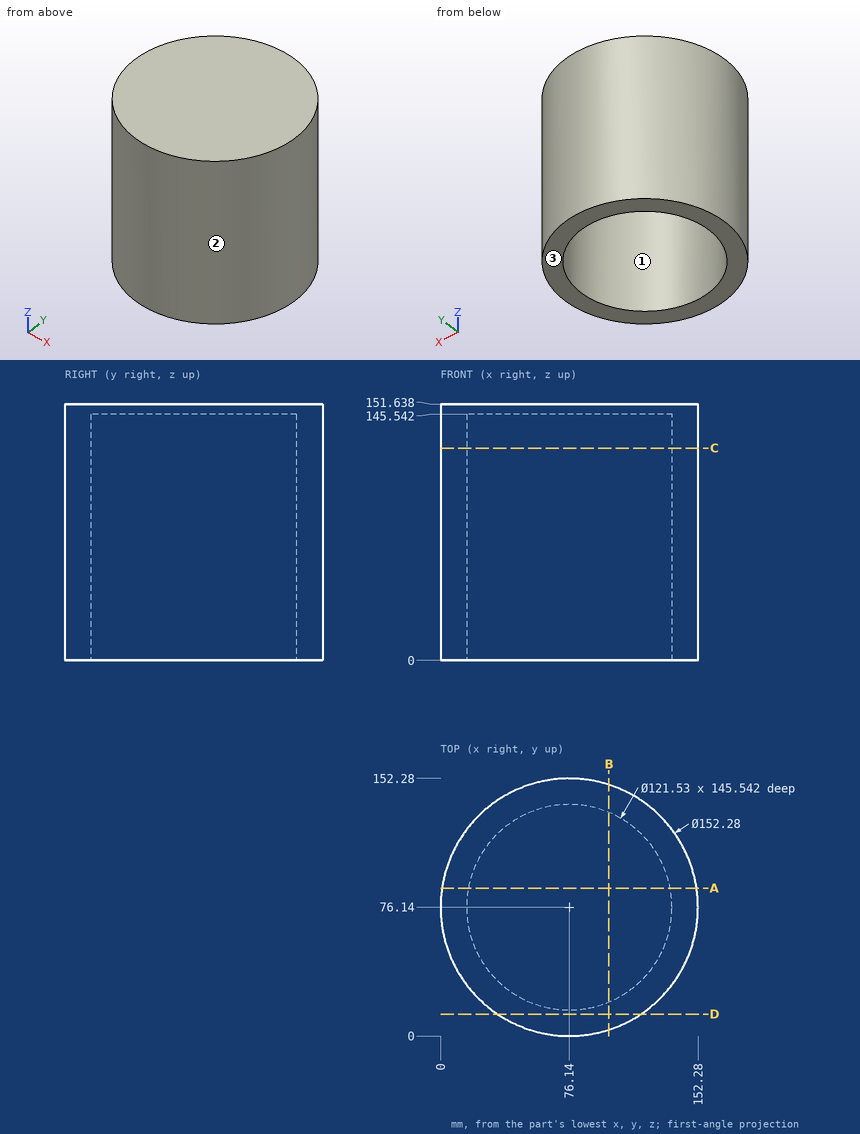
For this review, use the dimensioned drawing (mm, ordinates from the lowest corner) and the shaded views. Round coordinates to 2 decimals unless told otherwise and drop trailing zeros. Order: outer loops, then holes, each group sorted by start corner. A loop starts at its lowest first (then second) coordinate and runs counter-clockwise, first axis right, second up. Notation, with made-up numbers: (27, 78) -> (71, 78) arc R31 ccw to (71, 104) -> close; hole circle Ø11 at (43.5, 46.25). An arc over 180 degrees is marked (long way). One line per item, written item: value. Start each with the question number.
Q1. Take a section at C-C (z = 125.5). Write out the cut boundary in (x, y) (1 decimal).
Q2. Take a section at A-A (y = 87.5). Write out the cut boundary in (x, z), and give its area (3 significant figures).
Q3. Take a section at D-D (y = 13). Write out the cut boundary in (x, z), and give its area (3 significant figures).
Q4. Wall thickness on line 1 (Z direction, x = 55, y = 85.5); line 2 (Y direction, x = 95.5, z = 144.5); line 3 (Y direction, x = 71, z = 84) (1 decimal): over which ranges is each line inside the solid? List them lowest first.
Q5. Mouldability with a two-part tool opening along X and no side actions: class the marked faces 1, 2 and 3 as released by +X, released by -X, zero draft, split by the parting line, or undercut.
Q6. Take a section at B-B (x = 99.5). Write out the cut boundary in (y, z) (1 decimal), and give its area (3 significant figures).
Q7. Clearance check with flat-ended pins moving along their axes: pin 1 Ø10 at (x, y) = (71, 27.5) entering from -Z; pin 2 Ø10 at (x, z) = (19.5, 75.5) entering from -Y; pin 3 Ø8 at (y, z) = (53, 78.5) entering from +X (1 decimal). State where each tip first meets the part, or that it passes through.
Reported:
1. outline: circle Ø152.3 at (76.1, 76.1); hole circle Ø121.5 at (76.1, 76.1)
2. outline: (0.85, 0) -> (16.45, 0) -> (16.45, 145.54) -> (135.83, 145.54) -> (135.83, 0) -> (151.43, 0) -> (151.43, 151.64) -> (0.85, 151.64) -> close
2. area: 5,460 mm2
3. outline: (33.59, 0) -> (118.69, 0) -> (118.69, 151.64) -> (33.59, 151.64) -> close
3. area: 12,900 mm2
4. line 1: z = 145.54 to 151.64
4. line 2: y = 2.5 to 18.54, 133.74 to 149.78
4. line 3: y = 0.2 to 15.6, 136.7 to 152.1
5. face 1: undercut
5. face 2: split by the parting line
5. face 3: zero draft
6. outline: (3.7, 0) -> (20, 0) -> (20, 145.5) -> (132.2, 145.5) -> (132.2, 0) -> (148.6, 0) -> (148.6, 151.6) -> (3.7, 151.6) -> close
6. area: 5,650 mm2
7. pin 1: stops at z = 145.54
7. pin 2: stops at y = 20.19
7. pin 3: stops at x = 149.8
